Can you work these out from the model? Positions are in its coordinate system, mm. Face numbers are marked on the shaded views. A direction names the side the tool comes from. Coordinates: 2 decimals unless noted, no trailing zeros. Loops run counter-clockwise (first coordinate to the right, second up) from the corner with the lowest first, then second, coordinate; pieces in that order, holes last.
```python
from build123d import *

# Parameters (mm, degrees)
SKICA1_R                 = 1.6
P_IDAT_VYSUNUT_M1_DEPTH  = 1.6
SKICA2_W                 = 12.7
SKICA2_H                 = 6.7
P_IDAT_VYSUNUT_M2_DEPTH  = 5.7
SKICA3_W                 = 10
SKICA3_H                 = 6.9
P_IDAT_VYSUNUT_M3_DEPTH  = 5.9
SKICA4_W                 = 8.8
SKICA4_H                 = 4.7
SKICA4_W_2               = 0.6
SKICA4_H_2               = 0.6
ODEBRAT_VYSUNUT_M1_DEPTH = 5.4
SKICA5_W                 = 1.25
SKICA5_H                 = 3
ODEBRAT_VYSUNUT_M2_DEPTH = 11.4
SKICA6_W                 = 1.75
SKICA6_H                 = 4
ODEBRAT_VYSUNUT_M3_DEPTH = 1
ZAOBLIT1_R               = 0.2
SKICA8_R                 = 1.08
ODEBRAT_VYSUNUT_M4_DEPTH = 5.7
P_IDAT_VYSUNUT_M4_DEPTH  = 2
SKICA16_W                = 0.6
SKICA16_H                = 3
P_IDAT_VYSUNUT_M5_DEPTH  = 3.2
SKICA17_W                = 2.6
SKICA17_H                = 2.4
ODEBRAT_VYSUNUT_M6_DEPTH = 12


with BuildPart() as part:
    # Skica1 → Přidat vysunutím1 (new body)
    with BuildSketch(Plane.XY):
        with BuildLine():
            Line((0, 3.5), (20, 3.5))
            ThreePointArc((20, 3.5), (23.5, 0), (20, -3.5))
            Line((20, -3.5), (16.5, -3.5))
            Line((16.5, -3.5), (16.5, -9.5))
            Line((16.5, -9.5), (3.5, -9.5))
            Line((3.5, -9.5), (3.5, -3.5))
            Line((3.5, -3.5), (0, -3.5))
            ThreePointArc((0, -3.5), (-3.5, 0), (0, 3.5))
        make_face()
        Circle(SKICA1_R, mode=Mode.SUBTRACT)
        with Locations((20, 0)):
            Circle(SKICA1_R, mode=Mode.SUBTRACT)
    extrude(amount=P_IDAT_VYSUNUT_M1_DEPTH)

    # Skica2 → Přidat vysunutím2 (add)
    with BuildSketch(Plane.XY.offset(1.6)):
        with Locations((10, 6.35)):
            Rectangle(SKICA2_W, SKICA2_H)
    extrude(amount=P_IDAT_VYSUNUT_M2_DEPTH)

    # Skica3 → Přidat vysunutím3 (add)
    with BuildSketch(Plane.XY.offset(1.6)):
        with Locations((10, -10.55)):
            Rectangle(SKICA3_W, SKICA3_H)
    extrude(amount=P_IDAT_VYSUNUT_M3_DEPTH)

    # Skica4 → Odebrat vysunutím1 (cut)
    with BuildSketch(Plane.XZ.offset(14)):
        with Locations((10, 4.55)):
            Rectangle(SKICA4_W, SKICA4_H)
        with Locations((10, 5.2)):
            Rectangle(SKICA4_W_2, SKICA4_H_2, mode=Mode.SUBTRACT)
        with Locations((7.46, 5.2)):
            Rectangle(SKICA4_W_2, SKICA4_H_2, mode=Mode.SUBTRACT)
        with Locations((12.54, 5.2)):
            Rectangle(SKICA4_W_2, SKICA4_H_2, mode=Mode.SUBTRACT)
    extrude(amount=-ODEBRAT_VYSUNUT_M1_DEPTH, mode=Mode.SUBTRACT)

    # Skica5 → Odebrat vysunutím2 (cut)
    with BuildSketch(Plane(origin=(15, 0, 0), x_dir=(0, 0, -1), z_dir=(1, 0, 0))):
        with Locations((-6.125, -12.5)):
            Rectangle(SKICA5_W, SKICA5_H)
    extrude(amount=-ODEBRAT_VYSUNUT_M2_DEPTH, mode=Mode.SUBTRACT)

    # Skica6 → Odebrat vysunutím3 (cut)
    with BuildSketch(Plane.XY.offset(7.5)):
        with Locations((12.205, -12)):
            Rectangle(SKICA6_W, SKICA6_H)
        with Locations((7.795, -12)):
            Rectangle(SKICA6_W, SKICA6_H)
    extrude(amount=-ODEBRAT_VYSUNUT_M3_DEPTH, mode=Mode.SUBTRACT)

    # Zaoblit1
    zaoblit1_edges = [part.edges().sort_by_distance(p)[0] for p in [
        (16.5, -3.5, 0.8),
        (16.5, -9.5, 0.8),
        (3.5, -9.5, 0.8),
        (3.5, -3.5, 0.8),
    ]]
    fillet(zaoblit1_edges, radius=ZAOBLIT1_R)

    # Skica8 → Odebrat vysunutím4 (cut)
    with BuildSketch(Plane(origin=(0, -2.8, 7.3), x_dir=(1, 0, 0), z_dir=(0, 0, -1))):
        with Locations(Location((6.72, -7.28, 0), (0, 0, 65.14949766))):
            Circle(SKICA8_R)
        with Locations(Location((13.28, -7.28, 0), (0, 0, 65.14949766))):
            Circle(SKICA8_R)
    extrude(amount=ODEBRAT_VYSUNUT_M4_DEPTH, mode=Mode.SUBTRACT)

    # Skica15 → Přidat vysunutím4 (add, symmetric)
    with BuildSketch(Plane.XY.offset(4.45)):
        with BuildLine():
            Line((4.15, 9.7), (15.877570704, 12.162837052))
            ThreePointArc((15.877570704, 12.162837052), (16.38053334, 12.435762524), (16.651496116, 12.939785241))
            ThreePointArc((16.651496116, 12.939785241), (18.195492273, 14.317249988), (19.959455422, 13.23569219))
            Line((19.959455422, 13.23569219), (19.773836138, 13.161224202))
            ThreePointArc((19.773836138, 13.161224202), (18.174243185, 14.114045924), (16.833517959, 12.822139302))
            ThreePointArc((16.833517959, 12.822139302), (16.571348331, 12.286093255), (16.05055336, 11.994801518))
            Line((16.05055336, 11.994801518), (5.123136532, 9.7))
            Line((5.123136532, 9.7), (4.15, 9.7))
        make_face()
    extrude(amount=P_IDAT_VYSUNUT_M4_DEPTH, both=True)

    # Skica16 → Přidat vysunutím5 (add)
    with BuildSketch(Plane.XY.offset(4.8)):
        with Locations((4.9, 1.5)):
            Rectangle(SKICA16_W, SKICA16_H)
        with Locations((10, 1.5)):
            Rectangle(SKICA16_W, SKICA16_H)
        with Locations((15.1, 1.5)):
            Rectangle(SKICA16_W, SKICA16_H)
    extrude(amount=-P_IDAT_VYSUNUT_M5_DEPTH)

    # Skica17 → Odebrat vysunutím6 (cut)
    with BuildSketch(Plane(origin=(15.4, 0, 0), x_dir=(0, 0, -1), z_dir=(1, 0, 0))):
        with Locations((-2.9, 1.8)):
            Rectangle(SKICA17_W, SKICA17_H)
    extrude(amount=-ODEBRAT_VYSUNUT_M6_DEPTH, mode=Mode.SUBTRACT)


solid = part.part
```
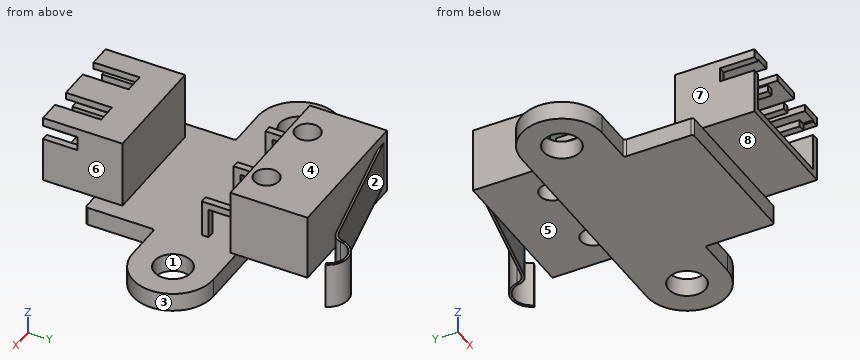
(1) I want a section at A-A on y = 4.48. Write out the boundary of the cut face in (x, z), then the cut area to 3 significant figures.
Check values:
outline: (3.65, 1.6) - (5.64, 1.6) - (5.64, 7.3) - (3.65, 7.3) - close; (7.8, 1.6) - (12.2, 1.6) - (12.2, 7.3) - (7.8, 7.3) - close; (14.36, 1.6) - (16.35, 1.6) - (16.35, 7.3) - (14.36, 7.3) - close
area: 47.8 mm2
(2) Which directions (+Z, -Z, +X, -X, +Y, -Y) give clear straight access to the entire face, cutting with the end or side of a thin tool? Please do the marked faces 4, 5, 6, 7 and 8.
Check values:
face 4: +Z, +X, -X, +Y
face 5: -Z, +X, -X, +Y
face 6: +Z, +X, -Y
face 7: +Z, -X, -Y
face 8: -Z, +X, -X, -Y
(3) If I drill on probe 1 along X at (y, z) = (4.48, 5.25); probe 2 along Z at (x, y) = (8.75, -9.75); probe 3 along Y at (x, z) = (13.28, 5.1), over which ranges is the centre line in solid material (lowest first)?
Check values:
probe 1: x = 3.65 to 5.64, 7.8 to 12.2, 14.36 to 16.35
probe 2: z = 1.6 to 2.2, 6.9 to 7.5
probe 3: y = -8.6 to -7.1, 3 to 3.4, 5.56 to 9.7, 11.41 to 11.62
(4) I want a section at B-B on x = 1. Write out the boundary of the cut face in (y, z), then the cut area to 3 significant figures.
Check values:
outline: (-3.5, 0) - (-1.25, 0) - (-1.25, 1.6) - (-3.5, 1.6) - close; (1.25, 0) - (3.5, 0) - (3.5, 1.6) - (1.25, 1.6) - close
area: 7.20 mm2
(5) If we mould it in two halves opening along Y, with no side actions, what happens to the marked faces 1, 2 and 3? For each: released by +Y, released by -Y, zero draft, split by the parting line, or undercut.
Check values:
face 1: undercut
face 2: released by +Y
face 3: split by the parting line
(6) I want a section at D-D on y = -4.25. Write out the boundary of the cut face in (x, z).
Check values:
outline: (3.5, 0) - (16.5, 0) - (16.5, 1.6) - (3.5, 1.6) - close
(7) I want a section at C-C on z = 1. Write out the boundary of the cut face in (x, y), then the cut area to 3 significant figures.
Check values:
outline: (0, -3.5) - (3.3, -3.5) arc R0.2 cw to (3.5, -3.7) - (3.5, -9.3) arc R0.2 ccw to (3.7, -9.5) - (16.3, -9.5) arc R0.2 ccw to (16.5, -9.3) - (16.5, -3.7) arc R0.2 cw to (16.7, -3.5) - (20, -3.5) arc R3.5 ccw to (20, 3.5) - (0, 3.5) arc R3.5 ccw to start; hole circle Ø3.2 at (0, 0); hole circle Ø3.2 at (20, 0)
area: 240 mm2
(8) I'm going to push flat-ended pins straight in: pin 1 (1.5 mm diameter, centred on x = 7, y = 5, fed in from +Z); pin 2 (0.5 mm diameter, centred on x = 12.5, y = -12, fed in from -Z); pin 3 (0.5 mm diameter, centred on y = -12, z = 5.5, fed in from -X). Where does each tip first touch, or does it pass through?
Check values:
pin 1: stops at z = 7.3
pin 2: stops at z = 1.6
pin 3: stops at x = 5
